Input: part model. Units: mm. Frame: model coordinates. Face numbers are marked on the shaded views. A direction names the side the tool comes from. Coordinates: 2 decimals unless noted, no trailing zeros. Write each loop counter-clockwise with the first axis right and the second up, starting at its lowest first coordinate (ties: lowest second). Pieces come first, ordered by that corner, then holes. Notation, with made-up numbers: (2, -30) - (7, -30) arc R12 cw to (7, -22) - close; hole circle Ø5 at (-29, -40). An arc over 180 degrees is marked (long way). One line per question, with ' | ' between items. Start each with the question number.
1) Section query A-A on z = -6. Return loops of the section in (x, y).
2) Section query B-B on x = 1. Return loops of the section in (y, z).
3) Reachability of the marked faces 4, 5 and 6 from +Z, -Z, +X, -X, +Y, -Y: full face, straight path, thin tool, end or side. Return the list, or none.
4) Line query: line 1 (Y direction, x = 4, z = -3); line 2 (Z direction, x = 8.75, y = 1.7); line 3 (X direction, y = 0.4, z = -8.75). Output: solid intervals per line, ascending.
5) First-contact query: P1, Ø1.5, axis at x = 6, y = 0.5, coming from the -Z side; P2, Ø0.8, axis at y = 1.5, z = -0.5, coming from the +X side; P3, Ø0.8, axis at x = 1.5, y = 1.5, coming from the -Z side. Flat tips, straight axial feed; report the tip coordinate or a pass-through.
6) Section query C-C on y = 1.35. Return loops of the section in (x, z).
7) Section query D-D on x = 3.75. Return loops of the section in (y, z).
8) Draft query along Z for the marked faces 1, 2 and 3. Return one class per face: released by +Z, released by -Z, zero draft, split by the parting line, or undercut.
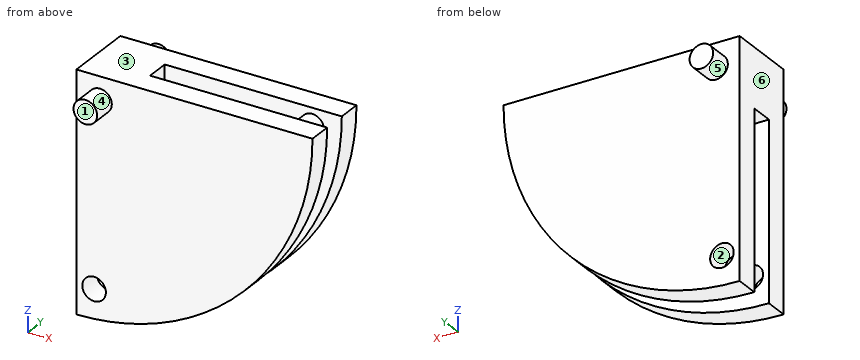
```python
from build123d import *

# Parameters (mm, degrees)
BOSS_EXTRUDE1_DEPTH      = 1
SKETCH2_R                = 0.5
SKETCH2_W                = 2.5
SKETCH2_H                = 2.5
BOSS_EXTRUDE2_DEPTH      = 1
BOSS_EXTRUDE3_DEPTH      = 1
SKETCH4_R                = 0.5
CUT_EXTRUDE1_DEPTH       = 15.456832295
BOSS_EXTRUDE4_DEPTH      = 1
BOSS_EXTRUDE4_DEPTH_BACK = 4
SKETCH5_R                = 0.5


with BuildPart() as part:
    # Sketch1 → Boss-Extrude1 (new body)
    with BuildSketch(Plane(origin=(0, 0, 0), x_dir=(1, 0, 0), z_dir=(0, 1, 0))):
        with BuildLine():
            Line((0, 0), (10, 0))
            ThreePointArc((10, 0), (7.071067812, 7.071067812), (0, 10))
            Line((0, 10), (0, 0))
        make_face()
    extrude(amount=BOSS_EXTRUDE1_DEPTH)

    # Sketch2 → Boss-Extrude2 (add)
    with BuildSketch(Plane(origin=(0, 1, 0), x_dir=(1, 0, 0), z_dir=(0, 1, 0))):
        with Locations(Location((8.75, 0.75, 0), (0, 0, 90))):
            Circle(SKETCH2_R)
        with Locations((1.25, 1.25)):
            Rectangle(SKETCH2_W, SKETCH2_H)
    extrude(amount=BOSS_EXTRUDE2_DEPTH)

    # Sketch3 → Boss-Extrude3 (add)
    with BuildSketch(Plane(origin=(0, 2, 0), x_dir=(1, 0, 0), z_dir=(0, 1, 0))):
        with BuildLine():
            Line((0, 10), (0, 0))
            Line((0, 0), (10, 0))
            ThreePointArc((10, 0), (7.071067812, 7.071067812), (0, 10))
        make_face()
    extrude(amount=BOSS_EXTRUDE3_DEPTH)

    # Sketch4 → Cut-Extrude1 (cut, through all)
    with BuildSketch(Plane(origin=(0, 3, 0), x_dir=(1, 0, 0), z_dir=(0, 1, 0))):
        with Locations(Location((0.75, 8.75, 0), (0, 0, 270))):
            Circle(SKETCH4_R)
    extrude(amount=-CUT_EXTRUDE1_DEPTH, mode=Mode.SUBTRACT)

    # Sketch5 → Boss-Extrude4 (add, two sides: drawn at the far end of the back side and taken through both)
    with BuildSketch(Plane(origin=(0, 3, 0), x_dir=(1, 0, 0), z_dir=(0, 1, 0)).offset(-BOSS_EXTRUDE4_DEPTH_BACK)):
        with Locations(Location((1, 1, 0), (0, 0, 270))):
            Circle(SKETCH5_R)
    extrude(amount=BOSS_EXTRUDE4_DEPTH + BOSS_EXTRUDE4_DEPTH_BACK)


solid = part.part
```
Answer key:
1) outline: (0, 0) - (8, 0) - (8, 1) - (0, 1) - close; (0, 2) - (8, 2) - (8, 3) - (0, 3) - close
2) outline: (-1, -1.5) - (0, -1.5) - (0, -8.32) - (1, -8.32) - (1, -2.5) - (2, -2.5) - (2, -8.32) - (3, -8.32) - (3, -1.5) - (4, -1.5) - (4, -0.5) - (3, -0.5) - (3, 0) - (0, 0) - (0, -0.5) - (-1, -0.5) - close; (0, -9.95) - (1, -9.95) - (1, -9.18) - (0, -9.18) - close; (2, -9.95) - (3, -9.95) - (3, -9.18) - (2, -9.18) - close
3) face 4: -Y | face 5: +Y | face 6: +Z, -Z, -X, +Y, -Y
4) line 1: 0 to 1, 2 to 3 | line 2: -1.25 to -0.25 | line 3: 0 to 0.25, 1.25 to 4.84
5) P1: z = -8.51 | P2: x = 9.25 | P3: z = -2.5
6) outline: (0, -2.5) - (2.5, -2.5) - (2.5, 0) - (0, 0) - close; circle Ø1 at (8.75, -0.75)
7) outline: (0, -9.27) - (1, -9.27) - (1, 0) - (0, 0) - close; (2, -9.27) - (3, -9.27) - (3, 0) - (2, 0) - close
8) face 1: zero draft | face 2: undercut | face 3: released by +Z
